from build123d import *

# Parameters (mm, degrees)
SKETCH020_W     = 400
SKETCH020_H     = 557.5
PAD008_DEPTH    = 12
SKETCH021_R     = 6.5
POCKET005_DEPTH = 12.001
SKETCH039_R     = 2.75
HOLE006_DEPTH   = 1386.241465


with BuildPart() as part:
    # Sketch020 → Pad008 (new body)
    with BuildSketch(Plane.XY):
        Rectangle(SKETCH020_W, SKETCH020_H)
    extrude(amount=PAD008_DEPTH)

    # Sketch021 → Pocket005 (cut, through all)
    with BuildSketch(Plane.XY):
        Circle(SKETCH021_R)
    extrude(amount=POCKET005_DEPTH, mode=Mode.SUBTRACT)

    # Sketch039 → Hole006 (cut)
    with BuildSketch(Plane.XY):
        with Locations((-24, 0)):
            Circle(SKETCH039_R)
        with Locations((24, 0)):
            Circle(SKETCH039_R)
    extrude(amount=HOLE006_DEPTH, mode=Mode.SUBTRACT)


solid = part.part
Input: part model. Units: mm. Frame: model coordinates. Give positions to 0.01 mm unless a question says otherwise; leave off trailing zeros. Order: outer loops, then holes, each group sorted by start corner. A loop starts at its lowest first (then second) coordinate and runs counter-clockwise, first axis right, second up.
Q1. Section A-A on x = 0. Output: boundary loops of the cut face in (y, z), and give its area (3 significant figures).
Checked values:
outline: (-278.75, 0) - (-6.5, 0) - (-6.5, 12) - (-278.75, 12) - close; (6.5, 0) - (278.75, 0) - (278.75, 12) - (6.5, 12) - close
area: 6,530 mm2
Q2. Ray query, probe 1 along X at (y, z) = (0, 9.75); probe 2 along Y at (x, z) = (0, 7.5); probe 3 along Y at (x, z) = (24, 6.5). Return the intervals inside material, ascending.
Checked values:
probe 1: x = -200 to -26.75, -21.25 to -6.5, 6.5 to 21.25, 26.75 to 200
probe 2: y = -278.75 to -6.5, 6.5 to 278.75
probe 3: y = -278.75 to -2.75, 2.75 to 278.75
Q3. Draft query along X for faces 1 (the flat face through (-3, -278.75, 6)), 2 (the flat face through (200, -4, 6)), 3 (the cylindrical face through (-5.158, -3.955, 5.916)). Return one class per face: +X half, -X half, draft (parallel to the pull), parting line (faces both ways), or undercut.
Checked values:
face 1: draft
face 2: +X half
face 3: undercut
